Part model, mm, in its own coordinate system. Face numbers are marked on the shaded views. Give positions to 0.01 mm unless a question says otherwise; leave off trailing zeros. Loops run counter-clockwise (first coordinate to the right, second up) from the corner with the lowest first, then second, coordinate; pieces in that order, holes last. Notation, with made-up numbers: M 64.25,86.25 L 92.25,86.25 A8 ccw 92.25,95.25 Z; hole C 75.5,67.25 d2. An arc over 180 degrees is marked long. Answer in a Markdown table with one row per item.
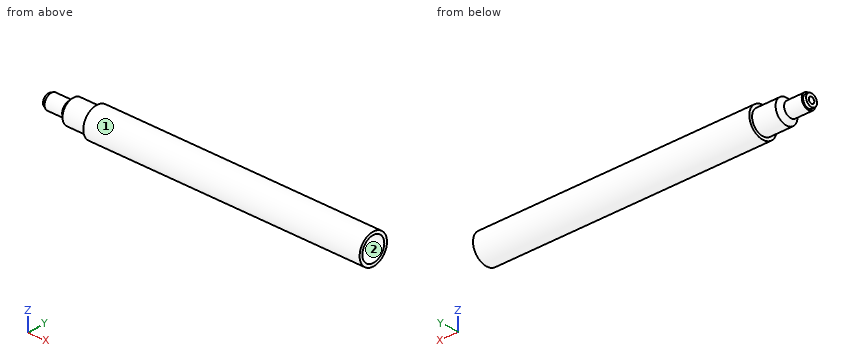
Autodesk Inventor part; units mm, degrees
ref_plane "YZ Plane" through (0, 0, 0) normal (1, 0, 0) x (0, 1, 0)
ref_plane "XZ Plane" through (0, 0, 0) normal (0, 1, 0) x (-1, 0, 0)
ref_plane "XY Plane" through (0, 0, 0) normal (0, 0, 1) x (1, 0, 0)
sketch "草图1" plane through (0, 0, 0) normal (1, 0, 0) x (0, 1, 0)
  circle A0 centre (0, 0) radius 5
  dimension "d0" = 10
extrude "body" add sketch "草图1" along normal blind 94
sketch "草图2" plane through (0, 0, 0) normal (0, 0, 1) x (1, 0, 0)
  line L0 (0, 0) -> (0, 4)
  line L1 (0, 5) -> (0, -5)
  line L2 (0, 4) -> (-2, 4)
  line L3 (-2, 4) -> (-4, 4)
  line L4 (-4, 4) -> (-8, 4)
  line L5 (-8, 4) -> (-9.5, 2.5)
  line L6 (-9.5, 2.5) -> (-15.5, 2.5)
  line L7 (-15.5, 2.5) -> (-15.5, 2)
  line L8 (-15.5, 2) -> (-16.5, 2)
  line L9 (-16.5, 2) -> (-16.5, 0)
  line L10 (-18.0565, 0) -> (1.4122, 0)
  line L11 (-16.5, 0) -> (0, 0)
  dimension "d3" = 4
  dimension "d4" = 2
  dimension "d5" = 2
  dimension "d6" = 4
  dimension "d9" = 1.5
  dimension "d10" = 1.5
  dimension "d11" = 6
  dimension "d12" = 0.5
  dimension "d13" = 1
revolve "旋转1" add sketch "草图2" angle 360 about axis through (-18.0565, 0, 0) along (1, 0, 0)
shell "抽壳1" thickness 1 removed faces 2 at (94, -0.591, 1.5584) at (-16.5, 0.343, 0.4805)
properties part number "pen"
(1) Pin check, flat tips, straight feed: pin 1 Ø5 at (y, z) = (0.5, 3.5) entering from +X; pin 2 Ø2.5 at (y, z) = (0, 0.5) entering from +X; pin 3 Ø6 at (x, z) = (33.5, 4) entering from +Y; pin 4 Ø2.5 at (y, z) = (0.5, -0.5) entering from +X. Stop position of each tip, or through.
Recorded:
| item | result |
|---|---|
| pin 1 | stops at x = 94 |
| pin 2 | stops at x = -8.84 |
| pin 3 | stops at y = 4.9 |
| pin 4 | stops at x = -8.63 |
(2) Drill centre lines: line 1 along Z through (x, y) = (-12.05, 0); line 2 along Z through (x, y) = (28, 0); line 3 along X through (y, z) = (-4, -1). Where is each one in solid material? Low to high.
Recorded:
| item | result |
|---|---|
| line 1 | z = -2.5 to -1.5, 1.5 to 2.5 |
| line 2 | z = -5 to -4, 4 to 5 |
| line 3 | x = 0 to 94 |
(3) Saw through at C-C (x = 79). Write the cut outline in (y, z), plus the area to 3 significant figures.
Recorded:
| item | result |
|---|---|
| outline | C 0,0 d10; hole C 0,0 d8 |
| area | 28.3 mm^2 |
(4) Pull direction Z, two halves, no side cores. Call the marked faces 1 and 2: +Z half, -Z half, draft (parallel to the pull), parting line (faces both ways), or undercut.
Recorded:
| item | result |
|---|---|
| face 1 | parting line |
| face 2 | undercut |
